For this review, take the finished solid that the model builds, in its own axes (mm). A direction names the side the tool comes from. Round coordinates to 2 decimals unless told otherwise and drop trailing zeros. Order: outer loops, then holes, each group sorted by start corner. A loop starts at its lowest first (then second) coordinate and runs counter-clockwise, first axis right, second up. Notation, with made-up numbers: (-35, -38) - (-31, -38) arc R15 ccw to (-31, -24) - close; hole circle Ø2 at (37, 8.25). An arc over 180 degrees is marked (long way). One line per question, with ' | ' between items.
```python
from build123d import *

# Parameters (mm, degrees)
SKETCH1_W           = 50.292
SKETCH1_H           = 50.292
BOSS_EXTRUDE1_DEPTH = 1.27
SKETCH1_3_W         = 53.292
SKETCH1_3_H         = 53.292
SKETCH1_3_W_2       = 50.292
SKETCH1_3_H_2       = 50.292
BOSS_EXTRUDE2_DEPTH = 11.43
SKETCH2_W           = 13.99999994
SKETCH2_H           = 10.16
CUT_EXTRUDE3_DEPTH  = 10
SKETCH3_W           = 9.5
SKETCH3_H           = 6.6
SKETCH3_W_2         = 5.1
SKETCH3_H_2         = 10.16
CUT_EXTRUDE4_DEPTH  = 10
SKETCH4_W           = 12.3
SKETCH4_H           = 10.16
CUT_EXTRUDE5_DEPTH  = 10
FILLET1_R           = 2.54
FILLET2_R           = 2.54
FILLET3_START       = -1
FILLET3_DEPTH       = 13
FILLET4_R           = 2.54
BOSS_EXTRUDE4_DEPTH = 3.048
HOLE1_D             = 3.0988
HOLE1_CBORE_D       = 5.461
HOLE1_CBORE_DEPTH   = 2.286


with BuildPart() as part:
    # Sketch1 → Boss-Extrude1 (new body)
    with BuildSketch(Plane(origin=(0, 0, 0), x_dir=(1, 0, 0), z_dir=(0, 1, 0))):
        Rectangle(SKETCH1_W, SKETCH1_H)
    extrude(amount=BOSS_EXTRUDE1_DEPTH)

    # Sketch1<3> → Boss-Extrude2 (add)
    with BuildSketch(Plane(origin=(0, 0, 0), x_dir=(1, 0, 0), z_dir=(0, 1, 0))):
        Rectangle(SKETCH1_3_W, SKETCH1_3_H)
        Rectangle(SKETCH1_3_W_2, SKETCH1_3_H_2, mode=Mode.SUBTRACT)
    extrude(amount=BOSS_EXTRUDE2_DEPTH)

    # Sketch2 → Cut-Extrude3 (cut)
    with BuildSketch(Plane.ZY.offset(26.646)):
        with Locations((-17.04600003, 6.35)):
            Rectangle(SKETCH2_W, SKETCH2_H)
    extrude(amount=-CUT_EXTRUDE3_DEPTH, mode=Mode.SUBTRACT)

    # Sketch3 → Cut-Extrude4 (cut)
    with BuildSketch(Plane.XY.offset(26.646)):
        with Locations((-19.356, 4.57)):
            Rectangle(SKETCH3_W, SKETCH3_H)
        with Locations((10.126, 6.35)):
            Rectangle(SKETCH3_W_2, SKETCH3_H_2)
    extrude(amount=-CUT_EXTRUDE4_DEPTH, mode=Mode.SUBTRACT)

    # Sketch4 → Cut-Extrude5 (cut)
    with BuildSketch(Plane(origin=(26.646, 0, 0), x_dir=(0, 0, -1), z_dir=(1, 0, 0))):
        with Locations((-18.996, 6.35)):
            Rectangle(SKETCH4_W, SKETCH4_H)
    extrude(amount=-CUT_EXTRUDE5_DEPTH, mode=Mode.SUBTRACT)

    # Fillet1
    fillet1_edges = [part.edges().sort_by_distance(p)[0] for p in [
        (26.646, 5.715, -26.646),
    ]]
    fillet(fillet1_edges, radius=FILLET1_R)

    # Fillet2
    fillet2_edges = [part.edges().sort_by_distance(p)[0] for p in [
        (-26.646, 5.715, -26.646),
    ]]
    fillet(fillet2_edges, radius=FILLET2_R)

    # Fillet3: read off the stored shape, not the designer's step
    # Fillet3 outline → Fillet3 (cut)
    with BuildSketch(Plane(origin=(0, 0, 0), x_dir=(1, 0, 0), z_dir=(0, 1, 0)).offset(FILLET3_START)):
        with BuildLine():
            Line((-26.646, -26.646), (-24.106, -26.646))
            ThreePointArc((-24.106, -26.646), (-25.902051224, -25.902051224), (-26.646, -24.106))
            Line((-26.646, -24.106), (-26.646, -26.646))
        make_face()
    extrude(amount=FILLET3_DEPTH, mode=Mode.SUBTRACT)

    # Fillet4
    fillet4_edges = [part.edges().sort_by_distance(p)[0] for p in [
        (26.646, 5.715, 26.646),
    ]]
    fillet(fillet4_edges, radius=FILLET4_R)

    # Sketch6 → Boss-Extrude4 (add)
    with BuildSketch(Plane(origin=(0, 1.27, 0), x_dir=(1, 0, 0), z_dir=(0, 1, 0))):
        with BuildLine():
            Line((26.646, -24.106), (26.646, 24.106))
            ThreePointArc((26.646, 24.106), (25.902051224, 25.902051224), (24.106, 26.646))
            Line((24.106, 26.646), (-24.106, 26.646))
            ThreePointArc((-24.106, 26.646), (-25.902051224, 25.902051224), (-26.646, 24.106))
            Line((-26.646, 24.106), (-26.646, -24.106))
            ThreePointArc((-26.646, -24.106), (-25.902051224, -25.902051224), (-24.106, -26.646))
            Line((-24.106, -26.646), (24.106, -26.646))
            ThreePointArc((24.106, -26.646), (25.902051224, -25.902051224), (26.646, -24.106))
        make_face()
    extrude(amount=-BOSS_EXTRUDE4_DEPTH)

    # Hole1 (through all)
    with Locations(Plane(origin=(-13.848520203, 1.27, 13.982017818), x_dir=(0, 0, 1), z_dir=(0, 1, 0))):
        with Locations((0, 0), (-27.830538021, -0.133497615), (-27.964035636, 27.697040406), (-0.133497615, 27.830538021)):
            CounterBoreHole(HOLE1_D / 2, HOLE1_CBORE_D / 2, HOLE1_CBORE_DEPTH)


solid = part.part
```
(1) For faces 1 (the flat face through (26.646, 5, -5)), 2 (the cylindrical face through (-12.137, 0.143, -15.861)), list the 3-axis set-ups (+Z, -Z, +X, -X, +Y, -Y) from which the entire face can be reached by the end or side of a thin tool; tool diameter is ignored.
Output values:
face 1: +Z, -Z, +X, +Y, -Y | face 2: +Y
(2) Mouldability with a two-part tool opening along Z and no side actions: class faces 3 (the flat face through (12.676, 6, 26)), 4 (the cylindrical face through (-12, 0.14, 11.97)), 5 (the cylindrical face through (25.922, 4.918, -25.882)) as released by +Z, released by -Z, zero draft, split by the parting line, or undercut.
Output values:
face 3: zero draft | face 4: undercut | face 5: released by -Z
(3) Insertion check: pin 1 (4.5 mm diameter, centred on x = -14.5, z = 14.5, fed in from +Y); pin 2 (1.2 mm diameter, centred on y = 3.5, z = 26, fed in from +X); pin 3 (1.2 mm diameter, centred on x = -26, y = 5.5, fed in from +Z). Each pin has a flat end and moves straight along its axis. Give the tip position at first contact, or say it passes through.
Output values:
pin 1: y = 1.27 | pin 2: x = 26.29 | pin 3: z = 26.29
(4) We need section B-B on x = -23. State the section outline as (y, z) points.
Output values:
outline: (-1.78, -26.65) - (11.43, -26.65) - (11.43, -25.15) - (1.27, -25.15) - (1.27, 26.65) - (-1.78, 26.65) - close; (7.87, 25.15) - (11.43, 25.15) - (11.43, 26.65) - (7.87, 26.65) - close
(5) We need section C-C on z = -13.5. State the section outline as (x, y) points.
Output values:
outline: (-26.65, -1.78) - (-15.49, -1.78) - (-15.49, -1.02) - (-16.69, -1.02) - (-16.69, 1.27) - (-26.65, 1.27) - close; (-12.47, -1.78) - (12.38, -1.78) - (12.38, -1.02) - (11.16, -1.02) - (11.16, 1.27) - (-11.27, 1.27) - (-11.27, -1.02) - (-12.47, -1.02) - close; (15.32, -1.78) - (26.65, -1.78) - (26.65, 11.43) - (25.15, 11.43) - (25.15, 1.27) - (16.54, 1.27) - (16.54, -1.02) - (15.32, -1.02) - close
(6) For probe 1 along X at (y, z) = (9.5, -8); probe 2 along Z at (x, y) = (12, -0.5), list the stretches that pass through material, from the lowest coordinate up. Write a range as [from, to].
Output values:
probe 1: [-26.65, -25.15], [25.15, 26.65] | probe 2: [-26.65, -15.99], [-11.97, 11.97], [15.73, 26.65]
(7) We need section D-D on x = 21. State the section outline as (y, z) points, plus the area to 3 significant figures.
Output values:
outline: (-1.78, -26.65) - (11.43, -26.65) - (11.43, -25.15) - (1.27, -25.15) - (1.27, 25.15) - (11.43, 25.15) - (11.43, 26.65) - (-1.78, 26.65) - close | area: 193 mm^2
(8) We need section A-A on y = 9.5. State the section outline as (x, z) points, plus the area to 3 significant figures.
Output values:
outline: (-26.65, -24.11) arc R2.54 ccw to (-24.11, -26.65) - (24.11, -26.65) arc R2.54 ccw to (26.65, -24.11) - (26.65, 12.85) - (25.15, 12.85) - (25.15, -25.15) - (-25.15, -25.15) - (-25.15, -24.05) - (-26.65, -24.05) - close; (-26.65, -10.05) - (-25.15, -10.05) - (-25.15, 25.15) - (7.58, 25.15) - (7.58, 26.65) - (-24.11, 26.65) arc R2.54 ccw to (-26.65, 24.11) - close; (12.68, 25.15) - (26.42, 25.15) arc R2.54 ccw to (24.11, 26.65) - (12.68, 26.65) - close | area: 258 mm^2
